Design review of the part built by this model. Coordinates are the model's own, in mm. Coordinates: 2 decimals unless noted, no trailing zeros. Write each loop counter-clockwise with the first axis right and the second up, starting at its lowest first coordinate (ties: lowest second). Pieces come first, ordered by that corner, then holes. Notation, with made-up numbers: (-32, -32) - (-26, -32) arc R23 ccw to (-26, -2) - close; hole circle Ø6 at (73.5, 31). An arc over 180 degrees is marked (long way). Use a Markdown table: item, result.
Autodesk Inventor part; units mm, degrees
ref_plane "YZ Plane" through (0, 0, 0) normal (1, 0, 0) x (0, 1, 0)
ref_plane "XZ Plane" through (0, 0, 0) normal (0, 1, 0) x (-1, 0, 0)
ref_plane "XY Plane" through (0, 0, 0) normal (0, 0, 1) x (1, 0, 0)
sketch "Esboço1" plane through (0, 0, 0) normal (0, 0, 1) x (1, 0, 0)
  line L0 (123.4, -20) -> (-123.4, -20)
  line L1 (-123.4, -20) -> (-123.4, 20)
  line L2 (-123.4, 20) -> (123.4, 20)
  line L3 (123.4, 20) -> (123.4, -20)
  line L4 (123.4, -20) -> (-123.4, 20) construction
  line L5 (-123.4, -20) -> (123.4, 20) construction
  line L6 (-123.4, -20) -> (-153.4, -20)
  line L7 (-153.4, -20) -> (-153.4, 0)
  line L8 (-153.4, 0) -> (-123.4, 0)
  line L9 (-123.4, 0) -> (-123.4, -20)
  line L10 (123.4, -20) -> (153.4, -20)
  line L11 (153.4, -20) -> (153.4, 0)
  line L12 (153.4, 0) -> (123.4, 0)
  line L13 (123.4, 0) -> (123.4, -20)
  point P0 (0, 0)
  dimension "d0" = 246.8
  dimension "d1" = 40
  dimension "d2" = 30
  dimension "d3" = 20
  dimension "d4" = 30
  dimension "d5" = 20
extrude "Placa1" add sketch "Esboço1" along normal blind 0.5
hole "Furo1" at (0, 5, 0.5) direction (0, 0, -1) diameter 4 depth 0.5 tip angle 118
hole "Furo2" at (-99, -13.5, 0.5) direction (0, 0, -1) diameter 3 depth 0.5 tip angle 118
hole "Furo3" at (99, -13.5, 0.5) direction (0, 0, -1) diameter 3 end through all
equation "\"d14\" = Espessura"
equation "\"d23\" = Espessura"
equation "\"d33\" = Espessura"
equation "\"d6\" = Espessura"
equation "\"Raio_vergadura\" = Espessura"
equation "\"Largura_alívio_de_vergadura\" = Espessura"
equation "\"Profundidade_alívio_de_vergadura\" = 0.5 * Espessura"
equation "\"Tamanho_alívio_de_dobra\" = 4 * Espessura"
equation "\"Remanescente_mínimo\" = 2 * Espessura"
equation "\"Raiodetransição\" = Raio_vergadura"
equation "\"Tamanho_de_raio_de_Jacobi\" = Raio_vergadura"
equation "\"TamanhoFolga\" = Espessura"
properties part number "Tampa Gaveta" material "PMMA plástico"
(1) Take a section at A-A on z = 0.2. Write out the cut boundary in (x, y), and give its area (3 significant figures).
Determined:
| item | result |
|---|---|
| outline | (-153.4, -20) - (153.4, -20) - (153.4, 0) - (123.4, 0) - (123.4, 20) - (-123.4, 20) - (-123.4, 0) - (-153.4, 0) - close; hole circle Ø3 at (-99, -13.5); hole circle Ø4 at (0, 5); hole circle Ø3 at (99, -13.5) |
| area | 11,000 mm2 |
(2) Take a section at B-B on x = 126. Write out the cut boundary in (y, z).
Determined:
| item | result |
|---|---|
| outline | (-20, 0) - (0, 0) - (0, 0.5) - (-20, 0.5) - close |
(3) For L1, parallel to X at y = -13.5, z = 0.45; L2, parallel to X at y = 5, z = 0.25; L3, parallel to Y at x = 99, z = 0.15, list the stretches that pass through material, from the lowest coordinate up. Write a range as from..to.
Determined:
| item | result |
|---|---|
| L1 | -153.4..-100.5, -97.5..97.5, 100.5..153.4 |
| L2 | -123.4..-2, 2..123.4 |
| L3 | -20..-15, -12..20 |
